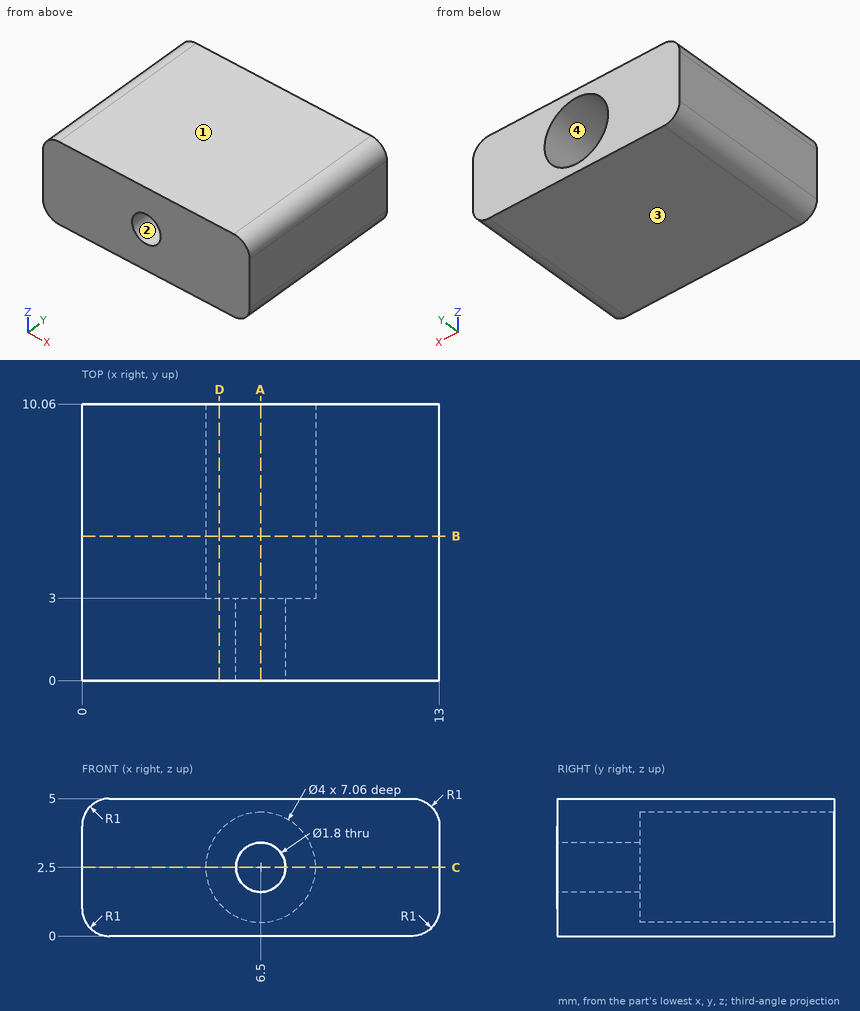
For this review, use the dimensioned drawing (mm, ordinates from the lowest corner) and the shaded views. Round coordinates to 2 decimals unless told otherwise and drop trailing zeros. Write each loop counter-clockwise with the first axis right and the second up, starting at its lowest first coordinate (ties: lowest second). Pieces come first, ordered by that corner, then holes. Notation, with made-up numbers: (35, 43.25) - (39, 43.25) arc R33 cw to (39, 75.25) - close; hole circle Ø7 at (4.5, -34). An arc over 180 degrees is marked (long way). Answer as a JSON object with one key per item and string values.
1. We need section D-D on x = 5. Give the boundary of the cut face in (y, z), then the cut area to 3 significant figures.
Response values:
{"outline": "(0, 0) - (10.06, 0) - (10.06, 1.18) - (3, 1.18) - (3, 3.82) - (10.06, 3.82) - (10.06, 5) - (0, 5) - close", "area": "31.6 mm2"}
2. Draft analysis for pull direction Z (two halves, no side actions). For the marked faces 1, 2, 3 and 4, state which applies: +Z half, -Z half, draft (parallel to the pull), parting line (faces both ways), or undercut.
Response values:
{"face 1": "+Z half", "face 2": "undercut", "face 3": "-Z half", "face 4": "undercut"}
3. We need section B-B on y = 5.25. Give the boundary of the cut face in (x, z), then the cut area to 3 significant figures.
Response values:
{"outline": "(0, 1) arc R1 ccw to (1, 0) - (12, 0) arc R1 ccw to (13, 1) - (13, 4) arc R1 ccw to (12, 5) - (1, 5) arc R1 ccw to (0, 4) - close; hole circle Ø4 at (6.5, 2.5)", "area": "51.6 mm2"}
4. We need section A-A on x = 6.5. Give the boundary of the cut face in (y, z).
Response values:
{"outline": "(0, 0) - (10.06, 0) - (10.06, 0.5) - (3, 0.5) - (3, 1.6) - (0, 1.6) - close; (0, 3.4) - (3, 3.4) - (3, 4.5) - (10.06, 4.5) - (10.06, 5) - (0, 5) - close"}
5. To check wall thickness, follow line 1 along Z through (x, y) = (6.5, 7.5); line 2 along Z through (x, y) = (6.5, 1.25); line 3 along X through (y, z) = (6, 2.5). State the ranges of each line that lie inside material, in increasing order.
Response values:
{"line 1": "z = 0 to 0.5, 4.5 to 5", "line 2": "z = 0 to 1.6, 3.4 to 5", "line 3": "x = 0 to 4.5, 8.5 to 13"}
6. We need section C-C on z = 2.5. Give the boundary of the cut face in (x, y), then the cut area to 3 significant figures.
Response values:
{"outline": "(0, 0) - (5.6, 0) - (5.6, 3) - (4.5, 3) - (4.5, 10.06) - (0, 10.06) - close; (7.4, 0) - (13, 0) - (13, 10.06) - (8.5, 10.06) - (8.5, 3) - (7.4, 3) - close", "area": "97.1 mm2"}
